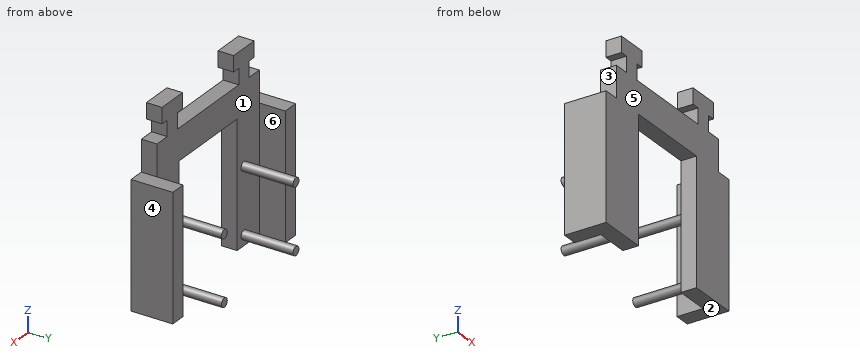
from build123d import *

# Parameters (mm, degrees)
BOSS_EXTRUDE1_DEPTH = 3
SKETCH2_R           = 0.85
SKETCH2_W           = 3
SKETCH2_H           = 24
BOSS_EXTRUDE2_DEPTH = 5
SKETCH3_R           = 0.85
BOSS_EXTRUDE3_DEPTH = 5


with BuildPart() as part:
    # Sketch1 → Boss-Extrude1 (new body)
    with BuildSketch(Plane(origin=(0, 0, 0), x_dir=(1, 0, 0), z_dir=(0, 1, 0))):
        Polygon((0, 0), (3, 0), (3, -3), (1.5, -3), (1.5, -6), (7.5, -6), (7.5, -3), (6, -3), (6, 0), (24, 0), (24, -3), (22.5, -3), (22.5, -6), (28.5, -6), (28.5, -3), (27, -3), (27, 0), (30, 0), (30, 6), (33, 6), (33, 30), (23.5, 30), (23.5, 6), (6.5, 6), (6.5, 30), (-3, 30), (-3, 6), (0, 6), align=None)
    extrude(amount=BOSS_EXTRUDE1_DEPTH)

    # Sketch2 → Boss-Extrude2 (add)
    with BuildSketch(Plane(origin=(0, 3, 0), x_dir=(1, 0, 0), z_dir=(0, 1, 0))):
        with Locations(Location((4.5, 28, 0), (0, 0, 270))):
            Circle(SKETCH2_R)
        with Locations(Location((25.5, 28, 0), (0, 0, 270))):
            Circle(SKETCH2_R)
        with Locations(Location((25.5, 15.5, 0), (0, 0, 270))):
            Circle(SKETCH2_R)
        with Locations(Location((4.5, 15.5, 0), (0, 0, 270))):
            Circle(SKETCH2_R)
        with Locations((-1.5, 18)):
            Rectangle(SKETCH2_W, SKETCH2_H)
        with Locations((31.5, 18)):
            Rectangle(SKETCH2_W, SKETCH2_H)
    extrude(amount=BOSS_EXTRUDE2_DEPTH)

    # Sketch3 → Boss-Extrude3 (add)
    with BuildSketch(Plane(origin=(0, 8, 0), x_dir=(1, 0, 0), z_dir=(0, 1, 0))):
        with Locations(Location((4.5, 28, 0), (0, 0, 270))):
            Circle(SKETCH3_R)
        with Locations(Location((25.5, 28, 0), (0, 0, 270))):
            Circle(SKETCH3_R)
        with Locations(Location((25.5, 15.5, 0), (0, 0, 270))):
            Circle(SKETCH3_R)
        with Locations(Location((4.5, 15.5, 0), (0, 0, 270))):
            Circle(SKETCH3_R)
    extrude(amount=BOSS_EXTRUDE3_DEPTH)


solid = part.part
Could you check a few things on this model? Use its own coordinates, in mm. Face numbers are marked on the shaded views. A direction names the side the tool comes from. Give positions to 0.01 mm unless a question says otherwise; leave off trailing zeros. Order: outer loops, then holes, each group sorted by start corner. A loop starts at its lowest first (then second) coordinate and runs counter-clockwise, first axis right, second up. Notation, with made-up numbers: (-24.5, 56) - (25.5, 56) arc R25 cw to (25.5, 74) - close; hole circle Ø5 at (-11.5, -16). An arc over 180 degrees is marked (long way). One line per question, with ' | ' between items. Start each with the question number.
Item 1: I want a section at A-A on z = -15.5. Write out the boundary of the cut face in (x, y), then the cut area to 3 significant figures.
Item 2: I want a section at D-D on z = -25. Write out the boundary of the cut face in (x, y), then the cut area to 3 significant figures.
Item 3: I need wall thicknesses on probe 1 along X at (y, z) = (7.75, -18); probe 2 along X at (y, z) = (2.5, -20); probe 3 along Z at (x, y) = (16, 1.25). Which ranges of each line are inside material? Lowest first, please. Write a range as [from, to].
Item 4: I want a section at B-B on y = 4.25. Write out the boundary of the cut face in (x, z).
Item 5: I want a section at C-C on x = 28. Write out the boundary of the cut face in (y, z), then the cut area to 3 significant figures.
Item 6: Thinking about a two-plate mould opening in X: for the marked faces 1, 2, 3 and 4, which applies, pulls with the +X half, pulls with the -X half, needs draft (parallel to the pull), parting line crosses it, or undercut?
Item 7: I'm going to push flat-ended pins straight in: pin 1 Ø1.5 at (y, z) = (2, 1) entering from -X; pin 2 Ø1.5 at (x, z) = (-1.5, -20) entering from +Y; pin 3 Ø2.5 at (y, z) = (1.5, 4) entering from -X. Where does each tip first touch, or does it pass through?
Item 8: For the marked faces 5 and 6, which set-ups out of +Z, -Z, +X, -X, +Y, -Y let a thin tool reach every point of the face, with its end or its side?
Verdict:
1) outline: (-3, 0) - (6.5, 0) - (6.5, 3) - (5.35, 3) - (5.35, 13) - (3.65, 13) - (3.65, 3) - (0, 3) - (0, 8) - (-3, 8) - close; (23.5, 0) - (33, 0) - (33, 8) - (30, 8) - (30, 3) - (26.35, 3) - (26.35, 13) - (24.65, 13) - (24.65, 3) - (23.5, 3) - close | area: 121 mm^2
2) outline: (-3, 0) - (6.5, 0) - (6.5, 3) - (0, 3) - (0, 8) - (-3, 8) - close; (23.5, 0) - (33, 0) - (33, 8) - (30, 8) - (30, 3) - (23.5, 3) - close | area: 87.0 mm^2
3) probe 1: [-3, 0], [30, 33] | probe 2: [-3, 6.5], [23.5, 33] | probe 3: [-6, 0]
4) outline: (-3, -30) - (0, -30) - (0, -6) - (-3, -6) - close; circle Ø1.7 at (4.5, -28); circle Ø1.7 at (4.5, -15.5); circle Ø1.7 at (25.5, -28); circle Ø1.7 at (25.5, -15.5); (30, -30) - (33, -30) - (33, -6) - (30, -6) - close
5) outline: (0, -30) - (3, -30) - (3, 0) - (0, 0) - close; (0, 3) - (3, 3) - (3, 6) - (0, 6) - close | area: 99.0 mm^2
6) face 1: undercut | face 2: needs draft | face 3: pulls with the -X half | face 4: pulls with the +X half
7) pin 1: x = 3 | pin 2: y = 8 | pin 3: x = 1.5
8) face 5: +Z, -Z, +X, -X, -Y | face 6: +Z, -Z, +Y
